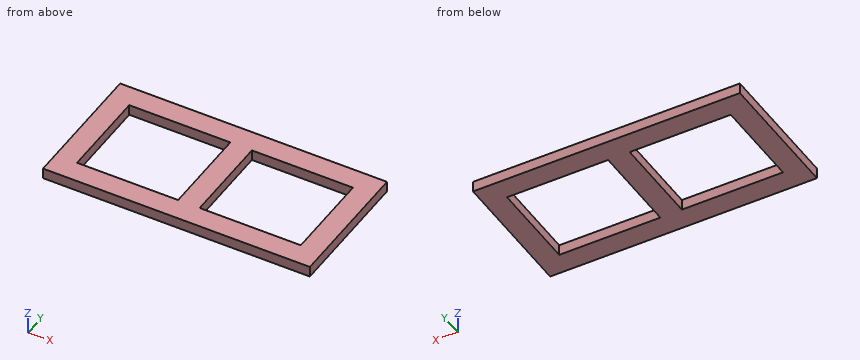
```python
from build123d import *

# Parameters (mm, degrees)
F0_W     = 1257.3
F0_H     = 628.65
F0_W_2   = 476.25
F0_H_2   = 425.45
F1_DEPTH = 25.4


with BuildPart() as f1:
    # F0 (on Top) → F1 (new body, symmetric)
    with BuildSketch(Plane.XY):
        Rectangle(F0_W, F0_H)
        with Locations((-288.925, 0)):
            Rectangle(F0_W_2, F0_H_2, mode=Mode.SUBTRACT)
        with Locations((288.925, 0)):
            Rectangle(F0_W_2, F0_H_2, mode=Mode.SUBTRACT)
    extrude(amount=F1_DEPTH, both=True)


solid = f1.part
```
CAD build for the part. Positions are in the model's coordinates, mm. Round coordinates to 2 decimals unless told otherwise and drop trailing zeros. Order: outer loops, then holes, each group sorted by start corner. A loop starts at its lowest first (then second) coordinate and runs counter-clockwise, first axis right, second up.
Q1. Slice it at A-A (x = -498). Write the cut outline in (y, z) (3 decimals), and give its area (3 significant figures).
Q2. Slice it at C-C (z = 5.5). Write the cut outline in (x, y) (3 decimals).
Q3. Slice it at B-B (y = 45.5). Write the cut outline in (x, z).
Q4. Wall check: L1, parallel to X at y = -75.5, z = 0; L2, parallel to Y at x = 316, z = -2 (3 decimals). Give the ranges that are in metal, low to high.
Results below:
1. outline: (-314.325, -25.4) - (-212.725, -25.4) - (-212.725, 25.4) - (-314.325, 25.4) - close; (212.725, -25.4) - (314.325, -25.4) - (314.325, 25.4) - (212.725, 25.4) - close
1. area: 10,300 mm2
2. outline: (-628.65, -314.325) - (628.65, -314.325) - (628.65, 314.325) - (-628.65, 314.325) - close; hole (-527.05, -212.725) - (-50.8, -212.725) - (-50.8, 212.725) - (-527.05, 212.725) - close; hole (50.8, -212.725) - (527.05, -212.725) - (527.05, 212.725) - (50.8, 212.725) - close
3. outline: (-628.65, -25.4) - (-527.05, -25.4) - (-527.05, 25.4) - (-628.65, 25.4) - close; (-50.8, -25.4) - (50.8, -25.4) - (50.8, 25.4) - (-50.8, 25.4) - close; (527.05, -25.4) - (628.65, -25.4) - (628.65, 25.4) - (527.05, 25.4) - close
4. L1: x = -628.65 to -527.05, -50.8 to 50.8, 527.05 to 628.65
4. L2: y = -314.325 to -212.725, 212.725 to 314.325
